```python
from build123d import *

# Parameters (mm, degrees)
SKIZZE1_W                       = 35
SKIZZE1_H                       = 26
AUFSATZ_LINEAR_AUSTRAGEN1_DEPTH = 8
AUFSATZ_LINEAR_AUSTRAGEN2_DEPTH = 3
SKIZZE3_R                       = 2.5
AUFSATZ_LINEAR_AUSTRAGEN3_DEPTH = 15
VERRUNDUNG1_R                   = 10


with BuildPart() as part:
    # Skizze1 → Aufsatz-Linear austragen1 (new body)
    with BuildSketch(Plane.XY):
        with Locations((0, -7)):
            Rectangle(SKIZZE1_W, SKIZZE1_H)
        Polygon((0, 2.5), (-2.5, 0), (0, -2.5), (2.5, 0), align=None, mode=Mode.SUBTRACT)
    extrude(amount=AUFSATZ_LINEAR_AUSTRAGEN1_DEPTH)

    # Skizze2 → Aufsatz-Linear austragen2 (add)
    with BuildSketch(Plane(origin=(0, 0, 0), x_dir=(-1, 0, 0), z_dir=(0, 0, -1))):
        Polygon((0, 6), (-4, 6), (-4, -20), (0, -20), (4, -20), (4, 6), align=None)
        Polygon((-2.5, 0), (0, -2.5), (2.5, 0), (0, 2.5), align=None, mode=Mode.SUBTRACT)
    extrude(amount=AUFSATZ_LINEAR_AUSTRAGEN2_DEPTH)

    # Skizze3 → Aufsatz-Linear austragen3 (add)
    with BuildSketch(Plane.XZ.offset(20)):
        with BuildLine():
            Line((0, 8), (-10, 8))
            Line((-10, 8), (-5.506451268, 18.383064085))
            ThreePointArc((-5.506451268, 18.383064085), (0, 22), (5.506451268, 18.383064085))
            Line((5.506451268, 18.383064085), (10, 8))
            Line((10, 8), (0, 8))
        make_face()
        with Locations((0, 16)):
            Circle(SKIZZE3_R, mode=Mode.SUBTRACT)
    extrude(amount=-AUFSATZ_LINEAR_AUSTRAGEN3_DEPTH)

    # Verrundung1
    verrundung1_edges = [part.edges().sort_by_distance(p)[0] for p in [
        (10, -12.5, 8),
        (-10, -12.5, 8),
    ]]
    fillet(verrundung1_edges, radius=VERRUNDUNG1_R)


solid = part.part
```
CAD build for the part. Positions are in the model's coordinates, mm. A direction names the side the tool comes from. Coordinates: 2 decimals unless noted, no trailing zeros. Loops run counter-clockwise (first coordinate to the right, second up) from the corner with the lowest first, then second, coordinate; pieces in that order, holes last. Notation, with made-up numbers: (2, 67) - (32, 67) arc R10 cw to (32, 78) - close; hole circle Ø8 at (-16, -24.5). An arc over 180 degrees is marked (long way). Return JSON: item names as keys, results as strings.
1. 3-axis set-ups, long thin cutter, end or side, ignore diameter. For faces 1 (the flat face through (-4, -7, -1)), 2 (the flat face through (0, -5, 12)), 3 (the flat face through (-17.5, -7, 4)), 4 (the flat face through (4, -7, -1)), 5 (the flat face through (-1.3, 1.2, 2.6)): which of +Z, -Z, +X, -X, +Y, -Y reach the whole face in a straight line?
Result:
{"face 1": "-Z, -X, +Y, -Y", "face 2": "+Z, +X, -X, +Y", "face 3": "+Z, -Z, -X, +Y, -Y", "face 4": "-Z, +X, +Y, -Y", "face 5": "+Z, -Z"}
2. Drop flat-ended pins along their axis: pin 1 (4 mm diameter, centred on x = -8.5, y = -13, fed in from -Z); pin 2 (2.5 mm diameter, centred on y = -4, z = -2, fed in from -X); pin 3 (3 mm diameter, centred on y = -12, z = 17, fed in from +X). Give the stop position or say it passes through.
Result:
{"pin 1": "stops at z = 0", "pin 2": "stops at x = -4", "pin 3": "stops at x = 6.75"}
3. Band-saw the part on A-A (y = 1). Give the cut face in (x, z), and give its area (3 significant figures).
Result:
{"outline": "(-17.5, 0) - (-4, 0) - (-4, -3) - (-1.5, -3) - (-1.5, 8) - (-17.5, 8) - close; (1.5, -3) - (4, -3) - (4, 0) - (17.5, 0) - (17.5, 8) - (1.5, 8) - close", "area": "271 mm2"}
4. Mould opens along Z. For faces 6 (the flat face through (6.436, -12.605, 16.236)), 7 (the flat face through (0, -7, -3)), 8 (the flat face through (1.3, -1.2, 2.6)), 9 (the cylindrical face through (-0.54, -12.6, 13.56)) say: released by +Z, released by -Z, zero draft, split by the parting line, or undercut.
Result:
{"face 6": "released by +Z", "face 7": "released by -Z", "face 8": "zero draft", "face 9": "undercut"}
5. Band-saw the part on B-B (z = 17.75). Give the cut face in (x, y).
Result:
{"outline": "(-5.78, -20) - (-1.79, -20) - (-1.79, -5) - (-5.78, -5) - close; (1.79, -20) - (5.78, -20) - (5.78, -5) - (1.79, -5) - close"}
6. Band-saw the part on D-D (x = -5). Give the cut face in (y, z), and give its area (3 significant figures).
Result:
{"outline": "(-20, 0) - (6, 0) - (6, 8) - (-5, 8) - (-5, 19.32) - (-20, 19.32) - close", "area": "378 mm2"}
7. Band-saw the part on C-C (y = -16). Give the cut face in (x, z).
Result:
{"outline": "(-17.5, 0) - (-4, 0) - (-4, -3) - (4, -3) - (4, 0) - (17.5, 0) - (17.5, 8) - (16.57, 8) arc R10 cw to (7.39, 14.03) - (5.51, 18.38) arc R6 ccw to (-5.51, 18.38) - (-7.39, 14.03) arc R10 cw to (-16.57, 8) - (-17.5, 8) - close; hole circle Ø5 at (0, 16)"}
8. Probe L1, parallel to X at y = 4.25, z = -0.75; L2, parallel to Y at x = -6, z = 11.25; L3, parallel to Z at x = 3, y = 1.25. List the from-to ranges inside material, lowest first. Write a range as from..to.
Result:
{"L1": "x = -4..4", "L2": "y = -20..-5", "L3": "z = -3..8"}
